The figure shows three views and two pictorial views of one solid part (mm, origin at its lowest corner). Answer the questions. A direction names the side the tool comes from. Coordinates: 2 decimals unless noted, no trailing zeros. Loops run counter-clockwise (first coordinate to the right, second up) from the corner with the lowest first, then second, coordinate; pieces in that order, holes last. Notation, with made-up numbers: (39.5, -37.5) - (73.5, -37.5) arc R33 ccw to (73.5, -1.5) - close; hole circle Ø6 at (54, 37.25). An arc over 180 degrees is marked (long way). Return JSON: item names as keys, results as strings. Group by question number.
1. Which of the six approach directions +Z, -Z, +X, -X, +Y, -Y give full straight-line access (tool end or side, diameter ignored) to the marked faces 4 and 5?
2. Find the intervals of material crossed by line 1 along X through (y, z) = (2.6, 10.05); line 2 along Y through (x, z) = (7.5, 13.75); line 3 along Z through (x, y) = (13.75, 2.2), in increasing order.
3. Section B-B (y = 2.4) is taken. Write down the section's boundary in (x, z), and give its area (3 significant figures).
4. The mould has two halves that part along X. Classify the marked faces 1, 2 and 3: pulls with the +X half, pulls with the -X half, needs draft (parallel to the pull), parting line crosses it, or undercut.
5. Section A-A (z = 10.05) is taken. Write down the section's boundary in (x, y).
6. Section D-D (z = 2) is taken. Write down the section's boundary in (x, y).
7. Each of these flat-tipped pins is pushed along its axis until it touches: P1, Ø3, axis at x = 8, z = 11, coming from the +Y side; P2, Ø2, axis at y = 2.5, z = 11.5, coming from the +X side; P3, Ø3, axis at x = 16, y = 0.5, coming from the +Z side. Where does it stop, or does it pass through?
8. Section C-C (x = 10.05) is taken. Write down the section's boundary in (y, z), and give its area (3 significant figures).
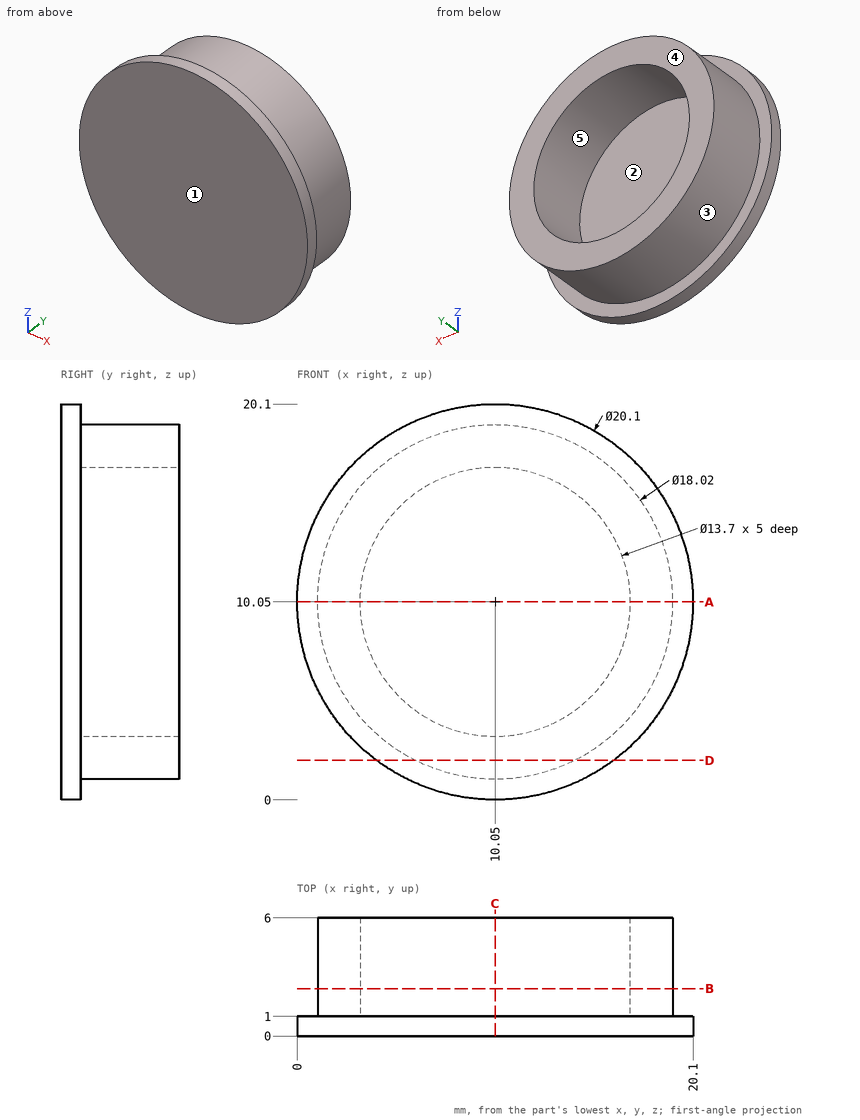
The answers:
{
 "1": {"face 4": "+Z, -Z, +X, -X, +Y", "face 5": "+Y"},
 "2": {"line 1": "x = 1.04 to 3.2, 16.9 to 19.06", "line 2": "y = 0 to 1", "line 3": "z = 1.83 to 4.29, 15.81 to 18.27"},
 "3": {"outline": "circle Ø18.02 at (10.05, 10.05); hole circle Ø13.7 at (10.05, 10.05)", "area": "108 mm2"},
 "4": {"face 1": "needs draft", "face 2": "undercut", "face 3": "parting line crosses it"},
 "5": {"outline": "(0, 0) - (20.1, 0) - (20.1, 1) - (19.06, 1) - (19.06, 6) - (16.9, 6) - (16.9, 1) - (3.2, 1) - (3.2, 6) - (1.04, 6) - (1.04, 1) - (0, 1) - close"},
 "6": {"outline": "(4.03, 0) - (16.07, 0) - (16.07, 1) - (14.1, 1) - (14.1, 6) - (6, 6) - (6, 1) - (4.03, 1) - close"},
 "7": {"P1": "stops at y = 1", "P2": "stops at x = 19.05", "P3": "stops at z = 19.06"},
 "8": {"outline": "(0, 0) - (1, 0) - (1, 1.04) - (6, 1.04) - (6, 3.2) - (1, 3.2) - (1, 16.9) - (6, 16.9) - (6, 19.06) - (1, 19.06) - (1, 20.1) - (0, 20.1) - close", "area": "41.7 mm2"}
}
